Part print with two shaded views. Sizes in mm from the minimum x, y, z corner. A direction names the side the tool comes from. Round coordinates to 2 decimals unless told otherwise and drop trailing zeros. Loops run counter-clockwise (first coordinate to the right, second up) from the corner with the lowest first, then second, coordinate; pieces in that order, holes last.
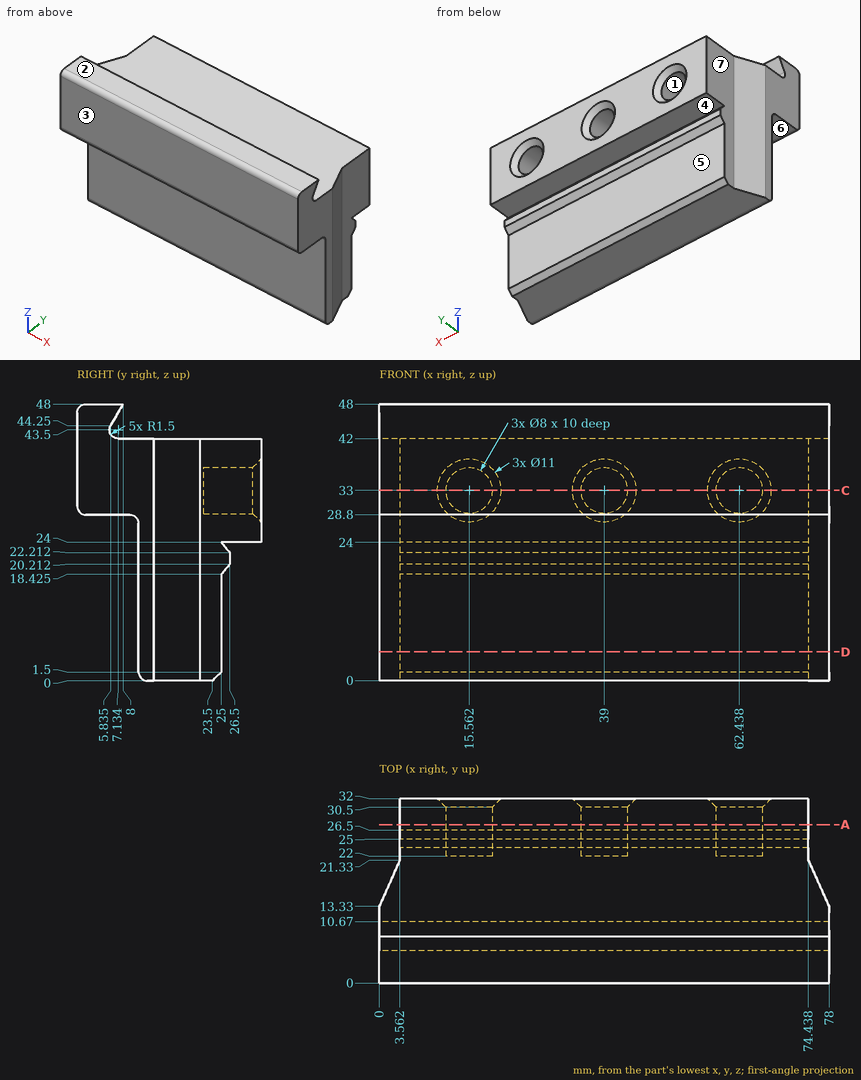
Item 1: Wall check: L1, parallel to Z at x = 39, y = 28; L2, parallel to Y at x = 45, z = 15.5; L3, parallel to Z at x = 68, y = 30. Give the ranges that are in metal, low to high.
Verdict:
L1: z = 24 to 29, 37 to 42
L2: y = 10.67 to 25
L3: z = 24 to 42
Item 2: Cut at D-D (z = 5). List the corners of the cut face in (x, y).
Verdict:
outline: (0, 10.67) - (78, 10.67) - (78, 13.33) - (74.44, 21.33) - (74.44, 25) - (3.56, 25) - (3.56, 21.33) - (0, 13.33) - close
Item 3: Cut at A-A (y = 27.5). List the corners of the cut face in (x, z).
Verdict:
outline: (3.56, 24) - (74.44, 24) - (74.44, 42) - (3.56, 42) - close; hole circle Ø8 at (15.56, 33); hole circle Ø8 at (39, 33); hole circle Ø8 at (62.44, 33)
Item 4: Cut at C-C (z = 33). List the corners of the cut face in (x, y), plus the area to 3 significant figures.
Verdict:
outline: (0, 0) - (78, 0) - (78, 13.33) - (74.44, 21.33) - (74.44, 32) - (67.94, 32) - (66.44, 30.5) - (66.44, 22) - (58.44, 22) - (58.44, 30.5) - (56.94, 32) - (44.5, 32) - (43, 30.5) - (43, 22) - (35, 22) - (35, 30.5) - (33.5, 32) - (21.06, 32) - (19.56, 30.5) - (19.56, 22) - (11.56, 22) - (11.56, 30.5) - (10.06, 32) - (3.56, 32) - (3.56, 21.33) - (0, 13.33) - close
area: 2,140 mm2
Item 5: Mould opens along Z. For the marked faces 1, 2 and 3 say: released by +Z, released by -Z, zero draft, split by the parting line, or undercut.
Verdict:
face 1: undercut
face 2: released by +Z
face 3: zero draft
Item 6: 3-axis set-ups, long thin cutter, end or side, ignore diameter. For the marked faces 4, 5, 6 and 7: which of +Z, -Z, +X, -X, +Y, -Y reach the whole face in a straight line?
Verdict:
face 4: +X, -X, +Y
face 5: -Z, +X, -X, +Y
face 6: -Z, +X, -X, -Y
face 7: +Z, -Z, -X, +Y
Item 7: Flat gauge pins, fed straight in: P1, Ø1.5, axis at y = 21.5, z = 5.5, coming from the +X side; P2, Ø12, axis at x = 48.5, z = 15.5, coming from the +Y side; P3, Ø6.5, axis at x = 41, z = 33, coming from the +Y side. Where does each tip first touch, or does it go through?
Verdict:
P1: stops at x = 74.7
P2: stops at y = 26.5
P3: stops at y = 31.75
